Verification items for the finished model (mm, model axes). Face numbers are marked on the shaded views. A direction names the side the tool comes from. Give positions to 0.01 mm unless a question says otherwise; leave off trailing zeros. Order: outer loops, then holes, each group sorted by start corner. A loop starts at its lowest first (then second) coordinate and runs counter-clockwise, first axis right, second up.
from build123d import *

# Parameters (mm, degrees)
SKETCH1_W            = 140
SKETCH1_H            = 76
BOSS_EXTRUDE1_DEPTH  = 45
FILLET2_R            = 10
CUT_EXTRUDE2_DEPTH   = 40
SKETCH5_W            = 40
SKETCH5_H            = 8
CUT_EXTRUDE3_DEPTH   = 2
FILLET3_R            = 5
FILLET3_OF_MIRROR1_R = 5
CHAMFER1_SIZE        = 0.5
CHAMFER1_SIZE2       = 0.866025404


with BuildPart() as part:
    # Sketch1 → Boss-Extrude1 (new body)
    with BuildSketch(Plane(origin=(0, 0, 0), x_dir=(1, 0, 0), z_dir=(0, 1, 0))):
        with Locations((70, 38)):
            Rectangle(SKETCH1_W, SKETCH1_H)
    extrude(amount=BOSS_EXTRUDE1_DEPTH)

    # Fillet2
    fillet2_edges = [part.edges().sort_by_distance(p)[0] for p in [
        (0, 22.5, -76),
        (140, 22.5, -76),
        (140, 22.5, 0),
        (0, 22.5, 0),
    ]]
    fillet(fillet2_edges, radius=FILLET2_R)

    # Sketch4 → Cut-Extrude2 (cut)
    with BuildSketch(Plane(origin=(0, 45, 0), x_dir=(1, 0, 0), z_dir=(0, 1, 0))):
        with BuildLine():
            Line((135, 10), (135, 66))
            ThreePointArc((135, 66), (133.535533906, 69.535533906), (130, 71))
            Line((130, 71), (10, 71))
            ThreePointArc((10, 71), (6.464466094, 69.535533906), (5, 66))
            Line((5, 66), (5, 10))
            ThreePointArc((5, 10), (6.464466094, 6.464466094), (10, 5))
            Line((10, 5), (130, 5))
            ThreePointArc((130, 5), (133.535533906, 6.464466094), (135, 10))
        make_face()
    extrude(amount=-CUT_EXTRUDE2_DEPTH, mode=Mode.SUBTRACT)

    # Sketch5 → Cut-Extrude3 (cut)
    with BuildSketch(Plane.XY):
        with Locations((70, 41)):
            Rectangle(SKETCH5_W, SKETCH5_H)
    cut_extrude3 = extrude(amount=-CUT_EXTRUDE3_DEPTH, mode=Mode.SUBTRACT)

    # Fillet3
    fillet3_edges = [part.edges().sort_by_distance(p)[0] for p in [
        (50, 37, -1),
        (90, 37, -1),
    ]]
    fillet(fillet3_edges, radius=FILLET3_R)

    # Mirror1: Cut-Extrude3 across plane
    add(cut_extrude3.mirror(Plane.XY.offset(-38)), mode=Mode.SUBTRACT)

    # Fillet3 of Mirror1
    fillet3_of_mirror1_edges = [part.edges().sort_by_distance(p)[0] for p in [
        (50, 37, -75),
        (90, 37, -75),
    ]]
    fillet(fillet3_of_mirror1_edges, radius=FILLET3_OF_MIRROR1_R)

    # Chamfer1
    chamfer1_edges = [part.edges().sort_by_distance(p)[0] for p in [
        (133.535533906, 45, -6.464466094),
        (135, 45, -38),
        (133.535533906, 45, -69.535533906),
        (70, 45, -71),
        (6.464466094, 45, -69.535533906),
        (5, 45, -38),
        (6.464466094, 45, -6.464466094),
        (70, 45, -5),
    ]]
    chamfer1_side = [part.faces().sort_by_distance(p)[0] for p in [
        (4.055342415, 45, -4.055342415),
    ]]
    chamfer(chamfer1_edges, length=CHAMFER1_SIZE, length2=CHAMFER1_SIZE2, reference=chamfer1_side[0])


solid = part.part
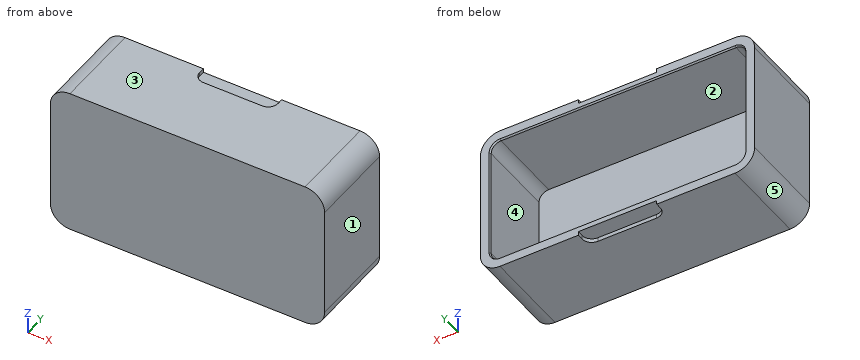
(1) Go/stop test with flat-tipped pins: pin 1 (2.5 mm diameter, centred on x = 73, y = 42, fed in from +Z); pin 2 (1 mm diameter, centred on y = 43.5, z = -75, fed in from -X); pin 3 (1 mm diameter, centred on y = 43.5, z = -0.5, fed in from +X). Record where each tip stops, or that it passes through.
Solved:
pin 1: stops at z = -2
pin 2: stops at x = 4.73
pin 3: stops at x = 134.36
(2) Section check C-C, the plane x = 118. Enter the section's corners in (y, z).
Solved:
outline: (0, -76) - (45, -76) - (45, -71.5) - (44.13, -71) - (5, -71) - (5, -5) - (44.13, -5) - (45, -4.5) - (45, 0) - (0, 0) - close
(3) Release check for a two-part mould opening along Z. For the marked faces 1, 2 and 3 record: pulls with the +Z half, pulls with the -Z half, needs draft (parallel to the pull), parting line crosses it, or undercut.
Solved:
face 1: needs draft
face 2: undercut
face 3: pulls with the +Z half
(4) Set-up check for the marked faces 4 and 5: record each of +Z, -Z, +X, -X, +Y, -Y from which the full face is reachable in a straight line by a thin tool's end or side.
Solved:
face 4: +Y
face 5: -Z, -X, +Y, -Y
(5) Section check A-A, the plane y = 29.5. Enter the section's corners in (x, z).
Solved:
outline: (0, -66) arc R10 ccw to (10, -76) - (130, -76) arc R10 ccw to (140, -66) - (140, -10) arc R10 ccw to (130, 0) - (10, 0) arc R10 ccw to (0, -10) - close; hole (5, -66) arc R5 ccw to (10, -71) - (130, -71) arc R5 ccw to (135, -66) - (135, -10) arc R5 ccw to (130, -5) - (10, -5) arc R5 ccw to (5, -10) - close
(6) Scan lines: line 1 (Z direction, x = 116, y = 19); line 2 (X direction, y = 40.5, z = -32.5); line 3 (Z direction, x = 60, y = 40.5). Record each from-to range of solid material in increasing order.
Solved:
line 1: z = -76 to -71, -5 to 0
line 2: x = 0 to 5, 135 to 140
line 3: z = -74 to -71, -5 to -2
(7) Section check B-B, the plane z = -32. Enter the section's corners in (x, y), then the cut area to 3 significant figures.
Solved:
outline: (0, 0) - (140, 0) - (140, 45) - (135.5, 45) - (135, 44.13) - (135, 5) - (5, 5) - (5, 44.13) - (4.5, 45) - (0, 45) - close
area: 1,100 mm2
(8) Section check D-D, the plane x = 78. Enter the section's corners in (y, z), then the cut area to 3 significant figures.
Solved:
outline: (0, -76) - (37, -76) - (37, -74) - (45, -74) - (45, -71.5) - (44.13, -71) - (5, -71) - (5, -5) - (44.13, -5) - (45, -4.5) - (45, -2) - (37, -2) - (37, 0) - (0, 0) - close
area: 748 mm2
